Read the model definition and answer for the solid it produces. Units are mm, in the model's axes. A direction names the side the tool comes from. Coordinates: 2 decimals unless noted, no trailing zeros. Loops run counter-clockwise (first coordinate to the right, second up) from the corner with the lowest first, then second, coordinate; pieces in that order, holes last. Notation, with made-up numbers: (-16, -32) - (25, -32) arc R21 ccw to (25, -7) - close; hole circle Ø6 at (32.5, 47). An arc over 180 degrees is marked (long way). One line per item, written item: value. Start each with the question number.
Autodesk Fusion 360 part; units mm, degrees
sketch "Lips" plane through (0, 0, 0) normal (0, 1, 0) x (1, 0, 0)
  circle A0 centre (0, 0) radius 17.05
  circle A1 centre (0, 0) radius 19.45
  dimension "d78" = 34.1
  dimension "d79" = 38.9
extrude "Lips (1)" add sketch "Lips" along normal blind 11.8 and the other way blind 8.2
sketch "Band" plane through (0, 0, 0) normal (0, 1, 0) x (1, 0, 0)
  circle A0 centre (0, 0) radius 17.05
  circle A1 centre (0, 0) radius 22
  dimension "d84" = 34.1
  dimension "d85" = 44
extrude "Band (1)" add sketch "Band" along normal blind 8.1941 and the other way blind 7.2
sketch "Outer cone profile" plane through (0, 0, 0) normal (0, 0, 1) x (1, 0, 0)
  line L0 (0, 1.75) -> (0, 22.5) construction
  line L1 (1.75, 0) -> (22.5, 0) construction
  line L2 (22, 5.6441) -> (22, 8.1941)
  line L3 (22, 8.1941) -> (19.45, 8.1941)
  line L4 (19.45, 8.1941) -> (22, 5.6441)
  dimension "d90" = 22
  dimension "d91" = 19.45
  dimension "d92" = 5.6441
  dimension "d93" = 8.1941
revolve "Outer cone" cut sketch "Outer cone profile" angle 360 about axis through (0, 1.75, 0) along (0, 1, 0)
sketch "Pocket profile" plane through (0, 0, 0) normal (0, 0, 1) x (1, 0, 0)
  line L0 (0, 1.75) -> (0, 22.5) construction
  line L1 (1.75, 0) -> (22.5, 0) construction
  line L2 (0, -7.2) -> (17.05, -7.2)
  line L3 (17.05, -7.2) -> (19.6, -4.65)
  line L4 (19.6, -4.65) -> (19.6, 4.65)
  line L5 (19.6, 4.65) -> (17.05, 7.2)
  line L6 (17.05, 7.2) -> (0, 7.2)
  line L7 (0, 7.2) -> (0, -7.2)
  dimension "d95" = 17.05
  dimension "d96" = 19.6
  dimension "d97" = 7.2
  dimension "d98" = 4.65
revolve "Pocket" cut sketch "Pocket profile" angle 360 about axis through (0, 1.75, 0) along (0, 1, 0)
sketch "Mouth" plane through (0, 0, 0) normal (0, 1, 0) x (1, 0, 0)
  line L0 (0, 0) -> (46.7654, -27)
  line L1 (46.7654, -27) -> (0, -54)
  line L2 (0, -54) -> (-46.7654, -27)
  line L3 (-46.7654, -27) -> (0, 0)
  line L4 (0, 0) -> (0, -54) construction
  dimension "d100" = 54
  dimension "d101" = 54
  dimension "d102" = 54
  dimension "d103" = 60
  dimension "d104" = 60
extrude "Mouth (1)" cut sketch "Mouth" along normal mid plane 30
ref_plane "WorkPlane3" through (0, 12.125, 0) normal (-0.1736, 0, -0.9848) x (0, 1, 0)
sketch "Stem slot section" plane through (0, 0, 0) normal (-0.1736, 0, -0.9848) x (0, 1, 0)
  line L0 (1.75, 0) -> (22.5, 0) construction
  line L1 (-4.65, 1.5) -> (4.65, 1.5)
  line L2 (4.65, 1.5) -> (4.65, -1.5)
  line L3 (4.65, -1.5) -> (-4.65, -1.5)
  line L4 (-4.65, -1.5) -> (-4.65, 1.5)
  line L5 (0, 0) -> (0, 4.8) construction
  dimension "d109" = 4.8
  dimension "d110" = 3
  dimension "d111" = 9.3
extrude "Stem slot" cut sketch "Stem slot section" along normal blind 6.4 from surface at 18.6
equation "rodOuterDiameter = 33.4 mm"
equation "collarClearance = 0.7 mm"
equation "collarWall = 2.4 mm"
equation "collarWidth = 20.0 mm"
equation "mouthHalfAngleDeg = 60.0 deg"
equation "ringOuterDiameter = 38.9 mm"
equation "ringWidth = 9.0 mm"
equation "stemThickness = 2.4 mm"
equation "stemAngleDeg = 100.0 deg"
equation "pocketClearance = 0.3 mm"
equation "slotClearance = 0.6 mm"
equation "pocketWidth = ringWidth + pocketClearance"
equation "pocketChamfer = ( ringOuterDiameter + pocketClearance ) / 2 - ( rodOuterDiameter + collarClearance ) / 2"
equation "bandWidth = pocketWidth + 2 * pocketChamfer"
equation "farLip = 1.0 mm"
equation "farExtent = bandWidth / 2 + farLip"
equation "chamferShift = collarWall * ( sqrt(2) - 1 )"
equation "d78 = rodOuterDiameter + collarClearance"
equation "d79 = rodOuterDiameter + collarClearance + 2 * collarWall"
equation "d80 = collarWidth - farExtent"
equation "d82 = farExtent"
equation "d84 = rodOuterDiameter + collarClearance"
equation "d85 = ringOuterDiameter + pocketClearance + 2 * collarWall"
equation "d86 = bandWidth / 2 + chamferShift"
equation "d88 = bandWidth / 2"
equation "d90 = ( ringOuterDiameter + pocketClearance + 2 * collarWall ) / 2"
equation "d91 = ( rodOuterDiameter + collarClearance + 2 * collarWall ) / 2"
equation "d92 = pocketWidth / 2 + chamferShift"
equation "d93 = bandWidth / 2 + chamferShift"
equation "d95 = ( rodOuterDiameter + collarClearance ) / 2"
equation "d96 = ( ringOuterDiameter + pocketClearance ) / 2"
equation "d97 = bandWidth / 2"
equation "d98 = pocketWidth / 2"
equation "d100 = Linear Dimension-2"
equation "d101 = Linear Dimension-3"
equation "d102 = Linear Dimension-4"
equation "d103 = mouthHalfAngleDeg"
equation "d104 = mouthHalfAngleDeg"
equation "d105 = collarWidth + 10 mm"
equation "d107 = stemAngleDeg"
equation "d109 = stemThickness * 2"
equation "d110 = stemThickness + slotClearance"
equation "d111 = pocketWidth"
equation "d112 = ( ringOuterDiameter + pocketClearance ) / 2 - 1 mm"
1) Section D-D, the plane y = 9.75 is taken. Determine the outline of the cut face in (x, z) (3 decimals).
2) Flat-ended cylindrical pins translate along their axes: P1, Ø3, axis at x = -4.5, z = -20, coming from the -Y side; P2, Ø1, axis at y = -6, z = -13, coming from the -X side; P3, Ø1.5, axis at x = 0.5, z = -16, coming from the +Y side; P4, Ø0.9, axis at x = -3, z = -20.5, coming from the +Y side. Find the tip coordinate at first contact, or state that the pin passes through.
3) Section C-C, the plane x = 0 is taken. Determine the outline of the cut face in (y, z).
4) Section A-A, the plane z = 0 is taken. Determine the outline of the cut face in (x, y).
5) Determine the mould class of faces 1 (the flat face through (-5.077, 0.065, -20.153)), 2 (the flat face through (-3, -8.2, -17)), 3 (the conical face through (-0.575, 8.035, -19.601)) for opening direction X: released by +X, released by -X, zero draft, split by the parting line, or undercut.
6) Straight lines are drawn through the part: L1, parallel to X at y = 10.25, z = 0; L2, parallel to X at y = -5, z = 10.5; L3, parallel to Z at x = -17.5, y = 1.25. For each, find the intervals that lie inside material, in ascending order.
7) For faces 4 (the conical face through (0.5, -7.04, -17.2)), 5 (the flat face through (-2.12, -0.07, -20.67)), 6 (the flat face through (17.355, 1.66, 10.02)), 7 (the cylindrical face through (0.57, -7.69, -19.44)), determine the directions among +Z, -Z, +X, -X, +Y, -Y from which every point of the face is accessible in a straight line to the end or side of a thin tool.
8) Section B-B, the plane y = 2.5 is taken. Determine the outline of the cut face in (x, z), and give its area (3 significant figures).
Answer below:
1. outline: (-16.844, 9.725) arc R19.45 ccw (long way) to (16.844, 9.725) - (14.766, 8.525) arc R17.05 cw (long way) to (-14.766, 8.525) - close
2. P1: y = -8.2
2. P2: x = -18.1
2. P3: through
2. P4: y = 7.38
3. outline: (-8.2, -19.45) - (-7.2, -19.45) - (-7.2, -22) - (5.64, -22) - (8.19, -19.45) - (11.8, -19.45) - (11.8, -17.05) - (7.2, -17.05) - (4.65, -19.6) - (-4.65, -19.6) - (-7.2, -17.05) - (-8.2, -17.05) - close
4. outline: (-22, -7.2) - (-19.45, -7.2) - (-19.45, -8.2) - (-17.05, -8.2) - (-17.05, -7.2) - (-19.6, -4.65) - (-19.6, 4.65) - (-17.05, 7.2) - (-17.05, 11.8) - (-19.45, 11.8) - (-19.45, 8.19) - (-22, 5.64) - close; (17.05, -8.2) - (19.45, -8.2) - (19.45, -7.2) - (22, -7.2) - (22, 5.64) - (19.45, 8.19) - (19.45, 11.8) - (17.05, 11.8) - (17.05, 7.2) - (19.6, 4.65) - (19.6, -4.65) - (17.05, -7.2) - close
5. face 1: undercut
5. face 2: zero draft
5. face 3: split by the parting line
6. L1: -19.45 to -17.05, 17.05 to 19.45
6. L2: -19.33 to -18.19, 18.19 to 19.33
6. L3: -13.33 to -8.83, 8.83 to 10.1
7. face 4: none
7. face 5: +Z
7. face 6: +Z, +Y, -Y
7. face 7: -Y
8. outline: (-19.05, 11) arc R22 ccw to (-5.29, -21.35) - (-4.87, -18.99) arc R19.6 cw to (-16.97, 9.8) - close; (-2.33, -21.88) arc R22 ccw to (19.05, 11) - (16.97, 9.8) arc R19.6 cw to (-1.92, -19.51) - close
8. area: 202 mm2
